```python
from build123d import *

# Parameters (mm, degrees)
F0_R     = 2.5
F1_DEPTH = 5


with BuildPart() as f1:
    # F0 (on Top) → F1 (new body)
    with BuildSketch(Plane.XY):
        with BuildLine():
            ThreePointArc((0, -5), (3.535534, -3.535534), (5, 0))
            Line((5, 0), (5, 15))
            ThreePointArc((5, 15), (0, 20), (-5, 15))
            ThreePointArc((-5, 15), (-7.928932, 7.928932), (-15, 5))
            ThreePointArc((-15, 5), (-20, 0), (-15, -5))
            Line((-15, -5), (0, -5))
        make_face()
        with Locations((-15, 0)):
            Circle(F0_R, mode=Mode.SUBTRACT)
        with Locations((0, 15)):
            Circle(F0_R, mode=Mode.SUBTRACT)
    extrude(amount=F1_DEPTH)


solid = f1.part
```
The listing builds one solid part. Answer for the finished solid, in the listing's coordinates (mm). Give positions to 0.01 mm unless a question says otherwise; leave off trailing zeros. Order: outer loops, then holes, each group sorted by start corner. A loop starts at its lowest first (then second) coordinate and runs counter-clockwise, first axis right, second up. Notation, with made-up numbers: (27.5, -19) -> (78.5, -19) arc R14 cw to (78.5, 0) -> close; hole circle Ø11 at (20, -8). An arc over 180 degrees is marked (long way). One line per item, written item: value.
1) Find section C-C, the plane y = 16.5. Determine the outline of the cut face in (x, z).
Reported:
outline: (-4.77, 0) -> (-2, 0) -> (-2, 5) -> (-4.77, 5) -> close; (2, 0) -> (4.77, 0) -> (4.77, 5) -> (2, 5) -> close
2) Find section A-A, the plane z = 1.65. Determine the outline of the cut face in (x, y), plus the area to 3 significant figures.
Reported:
outline: (-15, -5) -> (0, -5) arc R5 ccw to (5, 0) -> (5, 15) arc R5 ccw to (-5, 15) arc R10 cw to (-15, 5) arc R5 ccw to start; hole circle Ø5 at (-15, 0); hole circle Ø5 at (0, 15)
area: 355 mm^2
3) Determine the mould class of faces 1 (the cylindrical face through (-17.5, 0.1, 2.5)), 2 (the flat face through (-5, 5, 0)), 3 (the flat face through (-8, -5, 2)) for opening direction Y: pulls with the +Y half, pulls with the -Y half, needs draft (parallel to the pull), parting line crosses it, or undercut.
Reported:
face 1: undercut
face 2: needs draft
face 3: pulls with the -Y half
4) Find the intervals of material crossed by line 1 (Y direction, x = 0, z = 1.3); line 2 (Y direction, x = 0.5, z = 2.4); line 3 (X direction, y = 13.75, z = 0.9), in increasing order.
Reported:
line 1: y = -5 to 12.5, 17.5 to 20
line 2: y = -4.97 to 12.55, 17.45 to 19.97
line 3: x = -5.08 to -2.17, 2.17 to 5
5) Find section B-B, the plane x = 1. Determine the outline of the cut face in (y, z).
Reported:
outline: (-4.9, 0) -> (12.71, 0) -> (12.71, 5) -> (-4.9, 5) -> close; (17.29, 0) -> (19.9, 0) -> (19.9, 5) -> (17.29, 5) -> close
6) Flat-ended cylindrical pins translate along their axes: P1, Ø6, axis at x = -16.5, y = 4.5, coming from the -Z side; P2, Ø4, axis at x = -15, y = 0, coming from the +Z side; P3, Ø3, axis at y = 4, z = 4, coming from the -X side. Find the tip coordinate at first contact, or state that the pin passes through.
Reported:
P1: stops at z = 0
P2: passes through
P3: stops at x = -19.33
7) Find section D-D, the plane y = 4. Determine the outline of the cut face in (x, z).
Reported:
outline: (-18, 0) -> (5, 0) -> (5, 5) -> (-18, 5) -> close
